from build123d import *

# Parameters (mm, degrees)
SKETCH1_R           = 3.5
BOSS_EXTRUDE1_DEPTH = 2


with BuildPart() as part:
    # Sketch1 → Boss-Extrude1 (new body)
    with BuildSketch(Plane.XY):
        with BuildLine():
            Line((-17.5, -20), (-32.04293994, -20))
            Line((-32.04293994, -20), (-32.04293994, 8.228064973))
            ThreePointArc((-32.04293994, 8.228064973), (0, 33.082488619), (32.04293994, 8.228064973))
            Line((32.04293994, 8.228064973), (32.04293994, -20))
            Line((32.04293994, -20), (17.5, -20))
            Line((17.5, -20), (17, -20))
            Line((17, -20), (17, 0))
            ThreePointArc((17, 0), (0, 17), (-17, 0))
            Line((-17, 0), (-17, -20))
            Line((-17, -20), (-17.5, -20))
        make_face()
        with Locations((-25, -12.5)):
            Circle(SKETCH1_R, mode=Mode.SUBTRACT)
        with Locations((25, -12.5)):
            Circle(SKETCH1_R, mode=Mode.SUBTRACT)
    extrude(amount=BOSS_EXTRUDE1_DEPTH)


solid = part.part
Could you check a few things on this model? Use its own coordinates, in mm. A direction names the side the tool comes from. Give positions to 0.01 mm unless a question says otherwise; leave off trailing zeros. Write each loop counter-clockwise with the first axis right and the second up, starting at its lowest first coordinate (ties: lowest second). Pieces come first, ordered by that corner, then holes. Notation, with made-up numbers: (38.25, -13) - (67.25, -13) arc R21 ccw to (67.25, -1) - close; hole circle Ø1 at (-17.75, 14.5). An arc over 180 degrees is marked (long way). Use CSV: the item, a comma, the result in double quotes. Start each with the question number.
Item 1: I want a section at C-C, the plane x = 25. Please give me the cut outline in (y, z).
Item 2: I want a section at D-D, the plane y = 10.5. Please give me the cut outline in (x, z), then the cut area to 3 significant figures.
Item 3: If we mould it in two halves opening along X, with no side actions, what happens to faces 3 (the face through (0, 19, 2)), 4 (the face through (26.615, -15.605, 0.986)), 5 (the face through (-0.611, 33.077, 0.986))? For each: pulls with the +X half, pulls with the -X half, needs draft (parallel to the pull), parting line crosses it, or undercut.
Item 4: I'm going to push flat-ended pins straight in: pin 1 (8 mm diameter, centred on x = 18.5, y = 8.5, fed in from -Z); pin 2 (6.5 mm diameter, centred on x = 25, y = -12.5, fed in from +Z). Where does each tip first touch, or does it pass through?
Item 5: If I drill on line 1 along X through (y, z) = (-15.5, 1.1); line 2 along X through (y, z) = (-16.5, 0.6); line 3 along X through (y, z) = (15.5, 1.45), over which ranges is the centre line in solid material (lowest first)?
Item 6: I want a section at B-B, the plane z = 1. Please give me the cut outline in (x, y).
Item 7: I want a section at A-A, the plane y = -11. Please give me the cut outline in (x, z).
Item 8: For faces 1 (the face through (0, 19, 0)), 2 (the face through (-17, -10, 1)), which set-ups out of +Z, -Z, +X, -X, +Y, -Y let a thin tool reach every point of the face, with its end or its side?
Findings:
1,outline,"(-20, 0) - (-16, 0) - (-16, 2) - (-20, 2) - close; (-9, 0) - (21.67, 0) - (21.67, 2) - (-9, 2) - close"
2,outline,"(-31.37, 0) - (-13.37, 0) - (-13.37, 2) - (-31.37, 2) - close; (13.37, 0) - (31.37, 0) - (31.37, 2) - (13.37, 2) - close"
2,area,"72.0 mm2"
3,face 3,"needs draft"
3,face 4,"undercut"
3,face 5,"parting line crosses it"
4,pin 1,"stops at z = 0"
4,pin 2,"passes through"
5,line 1,"x = -32.04 to -26.8, -23.2 to -17, 17 to 23.2, 26.8 to 32.04"
5,line 2,"x = -32.04 to -17, 17 to 32.04"
5,line 3,"x = -29.23 to -6.98, 6.98 to 29.23"
6,outline,"(-32.04, -20) - (-17, -20) - (-17, 0) arc R17 cw to (17, 0) - (17, -20) - (32.04, -20) - (32.04, 8.23) arc R33.08 ccw to (-32.04, 8.23) - close; hole circle Ø7 at (-25, -12.5); hole circle Ø7 at (25, -12.5)"
7,outline,"(-32.04, 0) - (-28.16, 0) - (-28.16, 2) - (-32.04, 2) - close; (-21.84, 0) - (-17, 0) - (-17, 2) - (-21.84, 2) - close; (17, 0) - (21.84, 0) - (21.84, 2) - (17, 2) - close; (28.16, 0) - (32.04, 0) - (32.04, 2) - (28.16, 2) - close"
8,face 1,"-Z, +X, -X, +Y, -Y"
8,face 2,"+Z, -Z, -Y"
